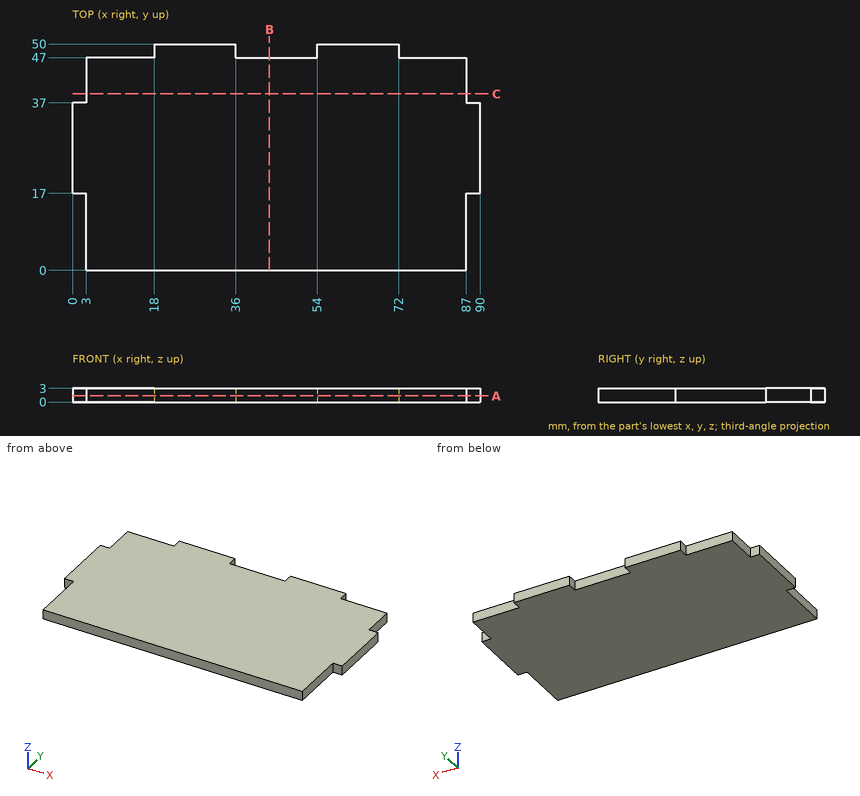
Part print with two shaded views. Sizes in mm from the minimum x, y, z corner. Give positions to 0.01 mm unless a question says otherwise; leave off trailing zeros. Order: outer loops, then holes, each group sorted by start corner. A loop starts at its lowest first (then second) coordinate and runs counter-clockwise, first axis right, second up. Notation, with made-up numbers: M 68.25,71 L 108.25,71 A23 ccw 108.25,81 Z; hole C -8,31.5 d6. An arc over 180 degrees is marked long. Use one line per item in the form item = value.
1) Probe probe 1 along X at (y, z) = (47.5, 1.45); probe 2 along X at (y, z) = (4, 0.45); probe 3 along Y at (x, z) = (82, 1.2). List the from-to ranges inside material, lowest first.
Calculated:
probe_1 = 18 to 36, 54 to 72
probe_2 = 3 to 87
probe_3 = 0 to 47
2) Saw through at B-B (x = 43.5). Give the cut face in (y, z).
Calculated:
outline = M 0,0 L 47,0 L 47,3 L 0,3 Z
3) Drop flat-ended pins along their axis: pin 1 (1.5 mm diameter, centred on y = 44, z = 1, fed in from +X); pin 2 (1.5 mm diameter, centred on y = 48.5, z = 2, fed in from +X); pin 3 (1.5 mm diameter, centred on x = 1.5, z = 2, fed in from -Y). Give the stop position or say it passes through.
Calculated:
pin_1 = 87
pin_2 = 72
pin_3 = 17
4) Saw through at A-A (z = 1.35). Give the cut face in (x, y).
Calculated:
outline = M 0,17 L 3,17 L 3,0 L 87,0 L 87,17 L 90,17 L 90,37 L 87,37 L 87,47 L 72,47 L 72,50 L 54,50 L 54,47 L 36,47 L 36,50 L 18,50 L 18,47 L 3,47 L 3,37 L 0,37 Z
5) Saw through at C-C (y = 39). Give the cut face in (x, z).
Calculated:
outline = M 3,0 L 87,0 L 87,3 L 3,3 Z
